Verification items for the finished model (mm, model axes). Face numbers are marked on the shaded views. A direction names the side the tool comes from. Round coordinates to 2 decimals unless told otherwise and drop trailing zeros. Write each loop counter-clockwise with the first axis right and the second up, starting at its lowest first coordinate (ties: lowest second). Pieces come first, ordered by that corner, then holes. Notation, with made-up numbers: (58.25, 14.25) - (62.25, 14.25) arc R12 cw to (62.25, 29.25) - close; hole circle Ø7 at (60, -13). An arc over 180 degrees is marked (long way). Write each question's results on one line, items separated by ' | '.
```python
from build123d import *

# Parameters (mm, degrees)
SKETCH_6_W          = 42.3
SKETCH_6_H          = 42.3
SKETCH_6_R          = 1.6
SKETCH_6_R_2        = 15
EXTRUDE_1_DEPTH     = 5
SKETCH_7_R          = 1.6
SKETCH_7_R_2        = 4.15
EXTRUDE_5_DEPTH     = 38
SKETCH_7_7_R        = 4.15
SKETCH_7_7_R_2      = 1.6
EXTRUDE_7_DEPTH     = 38
SKETCH_7_8_R        = 4.15
SKETCH_7_8_R_2      = 1.6
EXTRUDE_8_DEPTH     = 38
SKETCH_12_W         = 2
SKETCH_12_H         = 44.3
EXTRUDE_11_DEPTH    = 38
SKETCH_14_W         = 44.3
SKETCH_14_H         = 2
EXTRUDE_12_DEPTH    = 38
SKETCH_15_W         = 2
SKETCH_15_H         = 42.3
EXTRUDE_13_DEPTH    = 38
SKETCH_17_W         = 20.286999771
SKETCH_17_H         = 45
SKETCH_17_W_2       = 22.63718559
SKETCH_17_H_2       = 42.177300538
CUT_EXTRUDE_1_DEPTH = 13.2
SKETCH_18_W         = 9
SKETCH_18_H         = 8
CUT_EXTRUDE_2_DEPTH = 123


with BuildPart() as part:
    # 草图6 → 凸台-拉伸1 (new body)
    with BuildSketch(Plane(origin=(0, 0, 0), x_dir=(1, 0, 0), z_dir=(0, 1, 0))):
        Rectangle(SKETCH_6_W, SKETCH_6_H)
        with Locations(Location((15.5, 15.5, 0), (0, 0, 270))):
            Circle(SKETCH_6_R, mode=Mode.SUBTRACT)
        with Locations(Location((-15.5, 15.5, 0), (0, 0, 270))):
            Circle(SKETCH_6_R, mode=Mode.SUBTRACT)
        with Locations(Location((-15.5, -15.5, 0), (0, 0, 270))):
            Circle(SKETCH_6_R, mode=Mode.SUBTRACT)
        with Locations(Location((15.5, -15.5, 0), (0, 0, 270))):
            Circle(SKETCH_6_R, mode=Mode.SUBTRACT)
        with Locations(Location((0, 0, 0), (0, 0, 270))):
            Circle(SKETCH_6_R_2, mode=Mode.SUBTRACT)
    extrude(amount=EXTRUDE_1_DEPTH)

    # 草图7 → 凸台-拉伸5 (add)
    with BuildSketch(Plane(origin=(0, 5, 0), x_dir=(1, 0, 0), z_dir=(0, 1, 0))):
        with BuildLine():
            Line((56.202269248, -43.478354795), (21.15, -10.142654247))
            Line((21.15, -10.142654247), (21.15, -21.15))
            Line((21.15, -21.15), (10.142654247, -21.15))
            Line((10.142654247, -21.15), (41, -53.596295528))
            Line((41, -53.596295528), (41, -65))
            Line((41, -65), (59, -65))
            Line((59, -65), (59, -50))
            ThreePointArc((59, -50), (58.271046585, -46.45179082), (56.202269248, -43.478354795))
        make_face()
        with Locations(Location((50, -62, 0), (0, 0, 270))):
            Circle(SKETCH_7_R, mode=Mode.SUBTRACT)
        with Locations(Location((50, -50, 0), (0, 0, 270))):
            Circle(SKETCH_7_R_2, mode=Mode.SUBTRACT)
        with BuildLine():
            Line((-41, -53.596295528), (-10.142654247, -21.15))
            Line((-10.142654247, -21.15), (-21.15, -21.15))
            Line((-21.15, -21.15), (-21.15, -10.142654247))
            Line((-21.15, -10.142654247), (-56.202269248, -43.478354795))
            ThreePointArc((-56.202269248, -43.478354795), (-58.271046585, -46.45179082), (-59, -50))
            Line((-59, -50), (-59, -65))
            Line((-59, -65), (-41, -65))
            Line((-41, -65), (-41, -53.596295528))
        make_face()
        with Locations(Location((-50, -62, 0), (0, 0, 270))):
            Circle(SKETCH_7_R, mode=Mode.SUBTRACT)
        with Locations(Location((-50, -50, 0), (0, 0, 270))):
            Circle(SKETCH_7_R_2, mode=Mode.SUBTRACT)
    extrude(amount=-EXTRUDE_5_DEPTH)


with BuildPart() as extrude_7_tool:
    # 草图7<7> → 凸台-拉伸7 (new body)
    with BuildSketch(Plane(origin=(0, 5, 0), x_dir=(1, 0, 0), z_dir=(0, 1, 0))):
        with Locations(Location((-50, -50, 0), (0, 0, 270))):
            Circle(SKETCH_7_7_R)
        with Locations(Location((50, -50, 0), (0, 0, 270))):
            Circle(SKETCH_7_7_R)
        with Locations(Location((50, -62, 0), (0, 0, 270))):
            Circle(SKETCH_7_7_R_2)
        with Locations(Location((-50, -62, 0), (0, 0, 270))):
            Circle(SKETCH_7_7_R_2)
    extrude(amount=EXTRUDE_7_DEPTH)


with BuildPart() as part_1:
    add(part.part)


with BuildPart() as part_2:
    # 凸台-拉伸7: joined with extrude_7_tool
    add(part_1.part.fuse(extrude_7_tool.part, tol=0.00001))


with BuildPart() as extrude_7_kept_piece:
    # of the separate pieces the step leaves, the one the design keeps (extrude_7_pieces_kept)
    add(part_2.part.solids().sort_by_distance((-10.142654247, 0, 21.15))[0])


with BuildPart() as extrude_8_tool:
    # 草图7<8> → 凸台-拉伸8 (new body)
    with BuildSketch(Plane(origin=(0, 5, 0), x_dir=(1, 0, 0), z_dir=(0, 1, 0))):
        with Locations(Location((-50, -50, 0), (0, 0, 270))):
            Circle(SKETCH_7_8_R)
        with Locations(Location((50, -50, 0), (0, 0, 270))):
            Circle(SKETCH_7_8_R)
        with Locations(Location((50, -62, 0), (0, 0, 270))):
            Circle(SKETCH_7_8_R_2)
        with Locations(Location((-50, -62, 0), (0, 0, 270))):
            Circle(SKETCH_7_8_R_2)
    extrude(amount=EXTRUDE_8_DEPTH)


with BuildPart() as extrude_7_kept_piece_1:
    add(extrude_7_kept_piece.part)


with BuildPart() as extrude_7_kept_piece_2:
    # 凸台-拉伸8: joined with extrude_8_tool
    add(extrude_7_kept_piece_1.part.fuse(extrude_8_tool.part, tol=0.00001))


with BuildPart() as extrude_8_kept_piece:
    # of the separate pieces the step leaves, the one the design keeps (extrude_8_pieces_kept)
    add(extrude_7_kept_piece_2.part.solids().sort_by_distance((-10.142654247, 0, 21.15))[0])

    # 草图12 → 凸台-拉伸11 (add)
    with BuildSketch(Plane(origin=(0, 5, 0), x_dir=(1, 0, 0), z_dir=(0, 1, 0))):
        with Locations((22.15, -1)):
            Rectangle(SKETCH_12_W, SKETCH_12_H)
    extrude(amount=-EXTRUDE_11_DEPTH)

    # 草图14 → 凸台-拉伸12 (add)
    with BuildSketch(Plane(origin=(0, 5, 0), x_dir=(1, 0, 0), z_dir=(0, 1, 0))):
        with Locations((-1, -22.15)):
            Rectangle(SKETCH_14_W, SKETCH_14_H)
    extrude(amount=-EXTRUDE_12_DEPTH)

    # 草图15 → 凸台-拉伸13 (add)
    with BuildSketch(Plane(origin=(0, 5, 0), x_dir=(1, 0, 0), z_dir=(0, 1, 0))):
        with Locations((-22.15, 0)):
            Rectangle(SKETCH_15_W, SKETCH_15_H)
    extrude(amount=-EXTRUDE_13_DEPTH)

    # 草图17 → 切除-拉伸1 (cut)
    with BuildSketch(Plane.XZ.offset(33)):
        with Locations((49.343499886, 42.5)):
            Rectangle(SKETCH_17_W, SKETCH_17_H)
        with Locations((-50.518592795, 44.367414657)):
            Rectangle(SKETCH_17_W_2, SKETCH_17_H_2)
    extrude(amount=-CUT_EXTRUDE_1_DEPTH, mode=Mode.SUBTRACT)

    # 草图18 → 切除-拉伸2 (cut)
    with BuildSketch(Plane(origin=(59, 0, 0), x_dir=(0, 0, -1), z_dir=(1, 0, 0))):
        with Locations((-60.5, -8)):
            Rectangle(SKETCH_18_W, SKETCH_18_H)
    extrude(amount=-CUT_EXTRUDE_2_DEPTH, mode=Mode.SUBTRACT)


solid = extrude_8_kept_piece.part
```
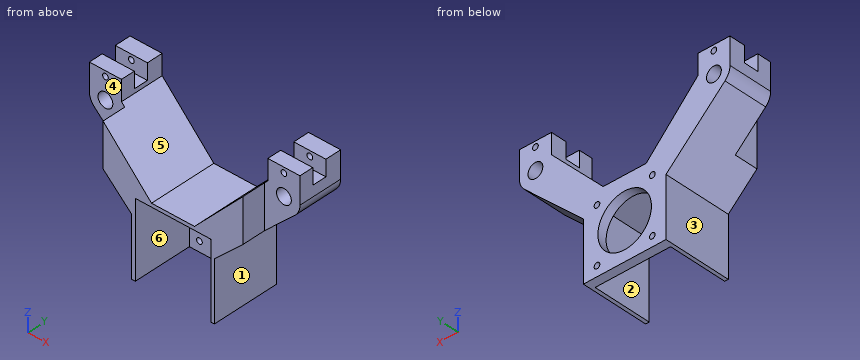
(1) Mould release check, pull along X, two halves, no side actions. Record for the marked faces 1, 2 and 3: released by +X, released by -X, zero draft, split by the parting line, or undercut.
Answer:
face 1: released by +X | face 2: undercut | face 3: released by -X
(2) Section check C-C (y = -14). Record the cut outline in (x, z), plus the area to 3 significant figures.
Answer:
outline: (-59, 50) arc R9 ccw to (-56.2, 43.48) - (-23.15, 12.04) - (-23.15, -21.15) - (-21.15, -21.15) - (-21.15, 21.15) - (21.15, 21.15) - (21.15, -21.15) - (23.15, -21.15) - (23.15, 12.04) - (56.2, 43.48) arc R9 ccw to (59, 50) - (59, 65) - (41, 65) - (41, 53.6) - (12.04, 23.15) - (-12.04, 23.15) - (-41, 53.6) - (-41, 65) - (-59, 65) - close; hole circle Ø8.3 at (-50, 50); hole circle Ø3.2 at (-50, 62); hole circle Ø8.3 at (50, 50); hole circle Ø3.2 at (50, 62) | area: 2,100 mm2
(3) Go/stop test with flat-tipped pins: pin 1 Ø16.5 at (y, z) = (-17.5, -0.5) entering from +X; pin 2 Ø3 at (x, z) = (-50, 62) entering from -Y; pin 3 Ø10.5 at (y, z) = (-27.5, 44.5) entering from -X; pin 4 Ø4.5 at (x, z) = (53, 60) entering from -Y. Record where each tip stops, or that it passes through.
Answer:
pin 1: x = 23.15 | pin 2: through | pin 3: x = -39.2 | pin 4: y = -19.8
(4) Section check A-A (z = 0). Record the cut outline in (x, y).
Answer:
outline: (-23.15, -33) - (-21.15, -33) - (-21.15, 0) - (-15, 0) - (-15, 5) - (-23.15, 5) - close; (15, 0) - (21.15, 0) - (21.15, -33) - (23.15, -33) - (23.15, 5) - (15, 5) - close
(5) Thickness scan on L1, parallel to X at y = -16, z = 62; L2, parallel to X at y = -15, z = 57; L3, parallel to X at y = -15, z = -1. Record the ranges inside material, lowest first.
Answer:
L1: -59 to -51.6, -48.4 to -41, 41 to 48.4, 51.6 to 59 | L2: -59 to -41, 41 to 59 | L3: -23.15 to -21.15, 21.15 to 23.15
(6) Section check D-D (z = 62). State how many separate pieces and enclosed holes the cut face has, plus the area to 3 significant figures.
Answer:
separate pieces: 8 | enclosed holes: 0 | area: 497 mm2
(7) Section check B-B (x = 0). Record the cut outline in (y, z).
Answer:
outline: (-33, 21.15) - (0, 21.15) - (0, 15) - (5, 15) - (5, 23.15) - (-33, 23.15) - close; (0, -21.15) - (5, -21.15) - (5, -15) - (0, -15) - close
(8) Set-up check for the marked faces 4, 5 and 6: record each of +Z, -Z, +X, -X, +Y, -Y from which the full face is reachable in a straight line by a thin tool's end or side.
Answer:
face 4: +Z, -Z, -X, -Y | face 5: +Z, +Y, -Y | face 6: -Z, -Y
